Work out the finished part from the listing and answer in its coordinate system (mm). A direction names the side the tool comes from. Round coordinates to 2 decimals unless told otherwise and drop trailing zeros. Write each loop counter-clockwise with the first axis right and the second up, starting at its lowest first coordinate (ties: lowest second). Pieces come first, ordered by that corner, then holes.
1. Find section A-A (y = 0). Write down the section's boundary in (x, z).
2. A tool of negligible diameter and unlimited length cuts with its end or side. For faces 4 (the face through (20, -48, 0)), 5 (the face through (0, -36, -24)), from which of +Z, -Z, +X, -X, +Y, -Y can it reach the whole face along a straight path? Write none if from no direction.
3. Straight lines are drawn through the part: probe 1 along Y at (x, z) = (8.25, 0); probe 2 along Y at (x, z) = (21.25, 0); probe 3 along Y at (x, z) = (11, 5.5). For each, find the intervals that lie inside material, in ascending order.
4. Flat-ended cylindrical pins translate along their axes: pin 1 Ø3.5 at (y, z) = (0, 48) entering from -X; pin 2 Ø1.5 at (x, z) = (17, -36) entering from +Y; pin 3 Ø4.5 at (y, z) = (-1.5, 48.5) entering from -X; pin 4 Ø3 at (x, y) = (24.5, 9.5) entering from -Z. Find the tip coordinate at first contact, or state that the pin passes through.
5. Determine the mould class of faces 1 (the face through (9.86, 45.267, 0.607)), 2 (the face through (30, 16, -40)), 3 (the face through (14.79, 16.16, -51.316)) for opening direction Z: pulls with the +Z half, pulls with the -Z half, needs draft (parallel to the pull), parting line crosses it, or undercut.
6. Find section C-C (x = 16). Write down the section's boundary in (y, z).
7. Find section D-D (z = 27). Write down the section's boundary in (x, y), and give its area (3 significant figures).
```python
from build123d import *

# Parameters (mm, degrees)
SKETCH1_R           = 53.8
SKETCH1_R_2         = 42.5
SKETCH1_R_3         = 2.8
BOSS_EXTRUDE1_DEPTH = 20
SKETCH3_R           = 53.8
SKETCH3_R_2         = 42.5
BOSS_EXTRUDE2_DEPTH = 10


with BuildPart() as part:
    # Sketch1 → Boss-Extrude1 (new body)
    with BuildSketch(Plane(origin=(0, 0, 0), x_dir=(0, 0, -1), z_dir=(1, 0, 0))):
        Circle(SKETCH1_R)
        Circle(SKETCH1_R_2, mode=Mode.SUBTRACT)
        with Locations((0, 48)):
            Circle(SKETCH1_R_3, mode=Mode.SUBTRACT)
        with Locations((48, 0)):
            Circle(SKETCH1_R_3, mode=Mode.SUBTRACT)
        with Locations((0, -48)):
            Circle(SKETCH1_R_3, mode=Mode.SUBTRACT)
        with Locations((-48, 0)):
            Circle(SKETCH1_R_3, mode=Mode.SUBTRACT)
    extrude(amount=BOSS_EXTRUDE1_DEPTH)

    # Sketch3 → Boss-Extrude2 (add)
    with BuildSketch(Plane(origin=(20, 0, 0), x_dir=(0, 0, -1), z_dir=(1, 0, 0))):
        Circle(SKETCH3_R)
        Circle(SKETCH3_R_2, mode=Mode.SUBTRACT)
    extrude(amount=BOSS_EXTRUDE2_DEPTH)


solid = part.part
```
Worked answers:
1. outline: (0, -53.8) - (30, -53.8) - (30, -42.5) - (0, -42.5) - (0, -45.2) - (20, -45.2) - (20, -50.8) - (0, -50.8) - close; (0, 42.5) - (30, 42.5) - (30, 53.8) - (0, 53.8) - (0, 50.8) - (20, 50.8) - (20, 45.2) - (0, 45.2) - close
2. face 4: -X
2. face 5: +Z, -Z, -X, +Y, -Y
3. probe 1: y = -53.8 to -50.8, -45.2 to -42.5, 42.5 to 45.2, 50.8 to 53.8
3. probe 2: y = -53.8 to -42.5, 42.5 to 53.8
3. probe 3: y = -53.52 to -42.14, 42.14 to 53.52
4. pin 1: stops at x = 20
4. pin 2: stops at y = 40.64
4. pin 3: stops at x = 0
4. pin 4: stops at z = -53.2
5. face 1: undercut
5. face 2: needs draft
5. face 3: parting line crosses it
6. outline: circle Ø107.6 at (0, 0); hole circle Ø5.6 at (-48, 0); hole circle Ø85 at (0, 0); hole circle Ø5.6 at (0, -48); hole circle Ø5.6 at (0, 48); hole circle Ø5.6 at (48, 0)
7. outline: (0, -46.53) - (30, -46.53) - (30, -32.82) - (0, -32.82) - close; (0, 32.82) - (30, 32.82) - (30, 46.53) - (0, 46.53) - close
7. area: 823 mm2
